CAD build for the part. Positions are in the model's coordinates, mm. A direction names the side the tool comes from. Coordinates: 2 decimals unless noted, no trailing zeros. Loops run counter-clockwise (first coordinate to the right, second up) from the corner with the lowest first, then second, coordinate; pieces in that order, holes last. Notation, with made-up numbers: (85, 1) - (140, 1) arc R31 cw to (140, 27) - close; hole circle Ø7 at (73.25, -39.5). An arc over 180 degrees is marked (long way). Put each result on its own line as item: value.
```python
from build123d import *

# Parameters (mm, degrees)
F0_W      = 609.6
F0_H      = 82.55
F1_DEPTH  = 12.7
F0_H_2    = 19.05
F1_FACE_W = 609.6
F1_FACE_H = 82.55
F2_DEPTH  = 12.7


with BuildPart() as f1:
    # F0 (on Top) → F1 (new body)
    with BuildSketch(Plane.XY):
        with Locations((-3.896274, 51.138431)):
            Rectangle(F0_W, F0_H)
    extrude(amount=F1_DEPTH)

    # F0 (on Top) + F1_face (on face) → F2 (join)
    with BuildSketch(Plane.XY):
        with Locations((-3.896274, 51.138431)):
            Rectangle(F0_W, F0_H)
        with Locations((-3.896274, 0.338431)):
            Rectangle(F0_W, F0_H_2)
    with BuildSketch(Plane(origin=(-3.896274, 51.138431, 12.7), x_dir=(1, 0, 0), z_dir=(0, 0, 1))):
        Rectangle(F1_FACE_W, F1_FACE_H)
    extrude(amount=F2_DEPTH)


solid = f1.part
```
Q1. Slice it at B-B, the plane z = 21. Give the cut face in (x, y).
Determined:
outline: (-308.7, 9.86) - (300.9, 9.86) - (300.9, 92.41) - (-308.7, 92.41) - close
Q2. Slice it at A-A, the plane x = -136.5. Give the cut face in (y, z), then the cut area to 3 significant figures.
Determined:
outline: (-9.19, 0) - (92.41, 0) - (92.41, 25.4) - (9.86, 25.4) - (9.86, 12.7) - (-9.19, 12.7) - close
area: 2,340 mm2
Q3. Tool access for faces 1 (the flat face through (-8, 52, 25.4)), 2 (the flat face through (-8, 0, 12.7)): list every direction of +Z, -Z, +X, -X, +Y, -Y with a clear straight run to the whole face (end or side of a thin tool).
Determined:
face 1: +Z, +X, -X, +Y, -Y
face 2: +Z, +X, -X, -Y
Q4. Wall check: L1, parallel to Y at x = -244.5, z = 16.5; L2, parallel to Z at x = -111, y = -3. Give the ranges that are in metal, low to high. Write a range as from..to.
Determined:
L1: 9.86..92.41
L2: 0..12.7
Q5. Pin check, flat tips, straight feed: pin 1 Ø5.5 at (x, y) = (89, -2.5) entering from +Z; pin 2 Ø4 at (x, z) = (-88.5, 19) entering from -Y. Stop position of each tip, or through.
Determined:
pin 1: z = 12.7
pin 2: y = 9.86
